Check sheet for the modelled part. Datum: model origin and axes. Units: mm. Round coordinates to 2 decimals unless told otherwise and drop trailing zeros. Write each loop counter-clockwise with the first axis right and the second up, starting at its lowest first coordinate (ties: lowest second). Pieces come first, ordered by that corner, then holes.
Item 1: Section check B-B, the plane z = 7.5. Record the cut outline in (x, y) (1 decimal).
Item 2: Depth check by flat-ended pin: pin 1 (4 mm diameter, centred on x = 47, z = 32.5, fed in from -Y); pin 2 (10 mm diameter, centred on x = -23.5, z = 178, fed in from +Y); pin 3 (6 mm diameter, centred on x = 65.5, y = -68.5, fed in from +Z). Enter the tip coordinate at first touch or a pass-through.
Item 3: Section check A-A, the plane z = 80.5. Record the cut outline in (x, y).
Item 4: Material ranges on line 1 along X through (y, z) = (67, 174.5); line 2 along Z through (x, y) = (-92.5, -2); line 3 along Z through (x, y) = (3, -28.5), recorded low to high.
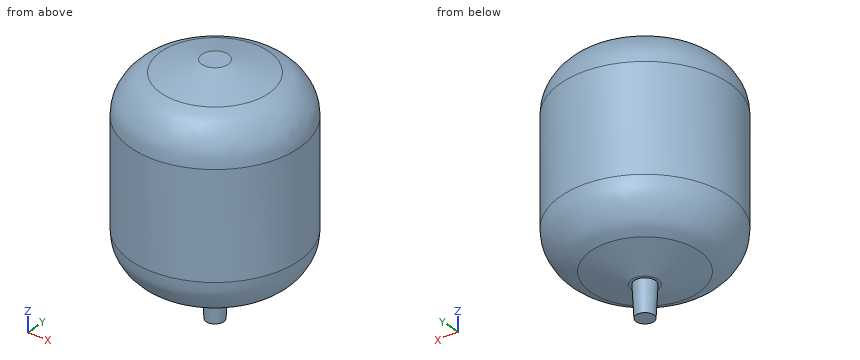
from build123d import *

# Parameters (mm, degrees)
F0_R     = 101.6
F1_DEPTH = 254
F2_R     = 12.7
F3_DEPTH = 38.1
F3_TAPER = 3
F4_SIZE2 = 85.725
F4_SIZE  = 25.4
F5_R     = 50.8


with BuildPart() as f1:
    # F0 (on Top) → F1 (new body)
    with BuildSketch(Plane.XY):
        Circle(F0_R)
    extrude(amount=F1_DEPTH)

    # F2 (on face) → F3 (join)
    with BuildSketch(Plane(origin=(0, 0, 0), x_dir=(1, 0, 0), z_dir=(0, 0, -1))):
        Circle(F2_R)
    extrude(amount=F3_DEPTH, taper=F3_TAPER)

    # F4
    f4_edges = [f1.edges().sort_by_distance(p)[0] for p in [
        (-101.6, 0, 254),
        (-101.6, 0, 0),
    ]]
    f4_side = f1.faces().sort_by_distance((-101.6, 0, 127))[0]
    chamfer(f4_edges, length=F4_SIZE, length2=F4_SIZE2, reference=f4_side)

    # F5
    f5_edges = [f1.edges().sort_by_distance(p)[0] for p in [
        (-101.6, 0, 25.4),
        (-101.6, 0, 228.6),
    ]]
    fillet(f5_edges, radius=F5_R)


solid = f1.part
Values found:
1. outline: circle Ø82.4 at (0, 0)
2. pin 1: stops at y = -80.19
2. pin 2: stops at y = 99.9
2. pin 3: stops at z = 220.7
3. outline: circle Ø203.2 at (0, 0)
4. line 1: x = -76.38 to 76.38
4. line 2: z = 34.35 to 219.65
4. line 3: z = 3.79 to 250.21
